Input: dimensioned drawing with shaded views. Units: mm. Origin: part minimum x, y, z. A direction names the side the tool comes from. Round coordinates to 2 decimals unless told otherwise and drop trailing zeros. Loops run counter-clockwise (first coordinate to the right, second up) from the corner with the lowest first, then second, coordinate; pieces in that order, holes last. Notation, with made-up numbers: (79.5, 20) - (111.5, 20) arc R25 cw to (111.5, 52) - close; hole circle Ø10 at (19, 3). An arc over 180 degrees is marked (long way). One line per question, with ' | ' between items.
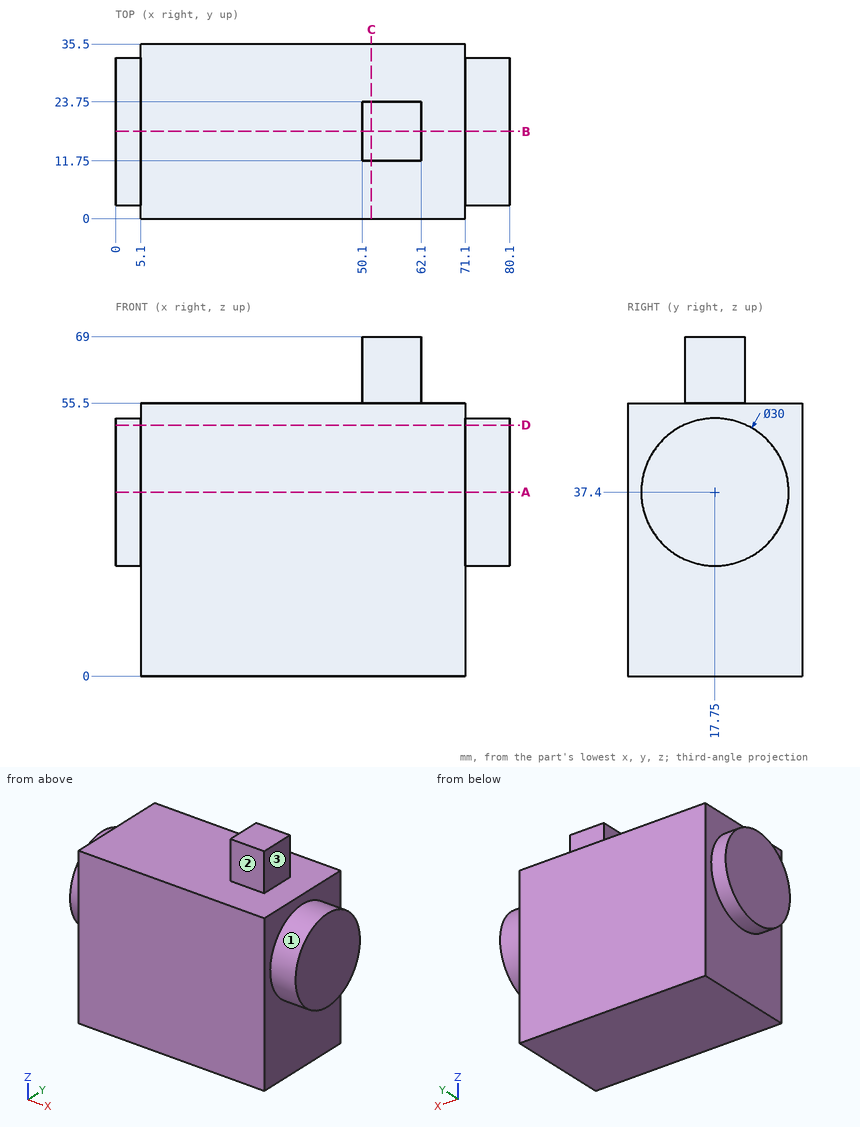
1. Section query D-D, the plane z = 51. Return loops of the section in (x, y), plus the area to 3 significant figures.
Worked out:
outline: (0, 11.42) - (5.1, 11.42) - (5.1, 0) - (71.1, 0) - (71.1, 11.42) - (80.1, 11.42) - (80.1, 24.08) - (71.1, 24.08) - (71.1, 35.5) - (5.1, 35.5) - (5.1, 24.08) - (0, 24.08) - close | area: 2,520 mm2
2. Access query for the marked faces 1, 2 and 3. Directions: +Z, -Z, +X, -X, +Y, -Y. A direction counts if a zero-diameter tool reaches every point of the face in a straight line with its end or side. Return the directions, or none.
Worked out:
face 1: +X | face 2: +Z, +X, -X, -Y | face 3: +Z, +X, +Y, -Y
3. Section query C-C, the plane x = 52. Return loops of the section in (y, z).
Worked out:
outline: (0, 0) - (35.5, 0) - (35.5, 55.5) - (23.75, 55.5) - (23.75, 69) - (11.75, 69) - (11.75, 55.5) - (0, 55.5) - close
4. Material intervals for probe 1 along X at (y, z) = (3.5, 44.5); probe 2 along Z at (x, y) = (58.5, 24); probe 3 along X at (y, z) = (20, 65), sorted ascending.
Worked out:
probe 1: x = 5.1 to 71.1 | probe 2: z = 0 to 55.5 | probe 3: x = 50.1 to 62.1
5. Section query A-A, the plane z = 37.4. Return loops of the section in (x, y), plus the area to 3 significant figures.
Worked out:
outline: (0, 2.75) - (5.1, 2.75) - (5.1, 0) - (71.1, 0) - (71.1, 2.75) - (80.1, 2.75) - (80.1, 32.75) - (71.1, 32.75) - (71.1, 35.5) - (5.1, 35.5) - (5.1, 32.75) - (0, 32.75) - close | area: 2,770 mm2
6. Contact query for flat-ended pins moving along their axis: P1, Ø12, axis at x = 19.5, y = 14, coming from the +Z side; P2, Ø6, axis at y = 20.5, z = 61.5, coming from the +X side; P3, Ø6, axis at y = 15.5, z = 60, coming from the -X side. Output: stop coordinate, or through.
Worked out:
P1: stops at z = 55.5 | P2: stops at x = 62.1 | P3: stops at x = 50.1
7. Section query B-B, the plane y = 17.75. Return loops of the section in (x, z).
Worked out:
outline: (0, 22.4) - (5.1, 22.4) - (5.1, 0) - (71.1, 0) - (71.1, 22.4) - (80.1, 22.4) - (80.1, 52.4) - (71.1, 52.4) - (71.1, 55.5) - (62.1, 55.5) - (62.1, 69) - (50.1, 69) - (50.1, 55.5) - (5.1, 55.5) - (5.1, 52.4) - (0, 52.4) - close
